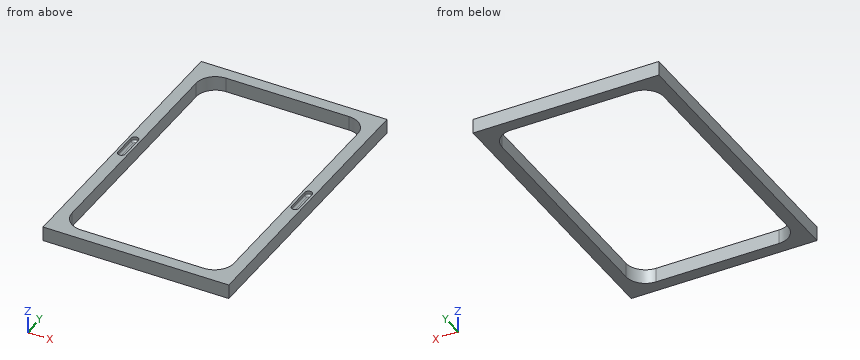
```python
from build123d import *

# Parameters (mm, degrees)
SKETCH1_W           = 977.9
SKETCH1_H           = 1524
BOSS_EXTRUDE1_DEPTH = 76.2
CUT_EXTRUDE1_DEPTH  = 25.4
FILLET1_R           = 10.16


with BuildPart() as part:
    # Sketch1 → Boss-Extrude1 (new body)
    with BuildSketch(Plane.XY):
        with Locations((488.95, 762)):
            Rectangle(SKETCH1_W, SKETCH1_H)
        with BuildLine():
            Line((63.5, 165.1), (63.5, 1358.9))
            ThreePointArc((63.5, 1358.9), (93.257951031, 1430.742048969), (165.1, 1460.5))
            Line((165.1, 1460.5), (812.8, 1460.5))
            ThreePointArc((812.8, 1460.5), (884.642048969, 1430.742048969), (914.4, 1358.9))
            Line((914.4, 1358.9), (914.4, 165.1))
            ThreePointArc((914.4, 165.1), (884.642048969, 93.257951031), (812.8, 63.5))
            Line((812.8, 63.5), (165.1, 63.5))
            ThreePointArc((165.1, 63.5), (93.257951031, 93.257951031), (63.5, 165.1))
        make_face(mode=Mode.SUBTRACT)
    extrude(amount=BOSS_EXTRUDE1_DEPTH)

    # Sketch2 → Cut-Extrude1 (cut)
    with BuildSketch(Plane.XY.offset(76.2)):
        with BuildLine():
            Line((50.8, 825.5), (50.8, 698.5))
            ThreePointArc((50.8, 698.5), (31.75, 679.45), (12.7, 698.5))
            Line((12.7, 698.5), (12.7, 825.5))
            ThreePointArc((12.7, 825.5), (31.75, 844.55), (50.8, 825.5))
        make_face()
        with BuildLine():
            Line((927.1, 825.5), (927.1, 698.5))
            ThreePointArc((927.1, 698.5), (946.15, 679.45), (965.2, 698.5))
            Line((965.2, 698.5), (965.2, 825.5))
            ThreePointArc((965.2, 825.5), (946.15, 844.55), (927.1, 825.5))
        make_face()
    extrude(amount=-CUT_EXTRUDE1_DEPTH, mode=Mode.SUBTRACT)

    # Fillet1
    fillet1_edges = [part.edges().sort_by_distance(p)[0] for p in [
        (31.75, 844.55, 50.8),
        (50.8, 762, 50.8),
        (31.75, 679.45, 50.8),
        (12.7, 762, 50.8),
        (946.15, 844.55, 50.8),
        (965.2, 762, 50.8),
        (946.15, 679.45, 50.8),
        (927.1, 762, 50.8),
    ]]
    fillet(fillet1_edges, radius=FILLET1_R)


solid = part.part
```
The model under review builds one solid part; all positions refer to its coordinate system, in mm. Round coordinates to 2 decimals unless told otherwise and drop trailing zeros. Loops run counter-clockwise (first coordinate to the right, second up) from the corner with the lowest first, then second, coordinate; pieces in that order, holes last. Notation, with made-up numbers: (22.5, 25.25) - (66.5, 25.25) arc R22 ccw to (66.5, 51.25) - close; hole circle Ø9 at (61.25, -17.5). An arc over 180 degrees is marked (long way). Use a Markdown table: item, result. Add a question column.
Q1. Add section B-B (x = 331.5). State the section outline as (y, z) points, plus the area to 3 significant figures.
Q2. Insertion check: pin 1 Ø12 at (y, z) = (776, 69.5) entering from -X; pin 2 Ø5.5 at (x, y) = (947, 794) entering from +Z. Each pin has a flat end and moves straight along its axis. Give the tip position at first contact, or say it passes through.
Q3. Add section A-A (y = 1017). State the section outline as (x, z) points, plus the area to 3 significant figures.
Q4. For probe 1 along Y at (x, z) = (330, 70.5); probe 2 along X at (y, z) = (1177.5, 4.5); probe 3 along Y at (x, z) = (159.5, 21.5), list the stretches that pass through material, from the lowest coordinate up.
Q5. Add section C-C (z = 27). State the section outline as (x, y) points, plus the area to 3 significant figures.
Worked answers:
| question | item | result |
|---|---|---|
| 1 | outline | (0, 0) - (63.5, 0) - (63.5, 76.2) - (0, 76.2) - close; (1460.5, 0) - (1524, 0) - (1524, 76.2) - (1460.5, 76.2) - close |
| 1 | area | 9,680 mm² |
| 2 | pin 1 | x = 0 |
| 2 | pin 2 | z = 50.8 |
| 3 | outline | (0, 0) - (63.5, 0) - (63.5, 76.2) - (0, 76.2) - close; (914.4, 0) - (977.9, 0) - (977.9, 76.2) - (914.4, 76.2) - close |
| 3 | area | 9,680 mm² |
| 4 | probe 1 | 0 to 63.5, 1460.5 to 1524 |
| 4 | probe 2 | 0 to 63.5, 914.4 to 977.9 |
| 4 | probe 3 | 0 to 63.65, 1460.35 to 1524 |
| 5 | outline | (0, 0) - (977.9, 0) - (977.9, 1524) - (0, 1524) - close; hole (63.5, 165.1) arc R101.6 ccw to (165.1, 63.5) - (812.8, 63.5) arc R101.6 ccw to (914.4, 165.1) - (914.4, 1358.9) arc R101.6 ccw to (812.8, 1460.5) - (165.1, 1460.5) arc R101.6 ccw to (63.5, 1358.9) - close |
| 5 | area | 310,000 mm² |
